Read the model definition and answer for the solid it produces. Units are mm, in the model's axes. A direction names the side the tool comes from. Give positions to 0.01 mm unless a question says otherwise; leave off trailing zeros. Loops run counter-clockwise (first coordinate to the right, second up) from the corner with the lowest first, then second, coordinate; pieces in that order, holes last. Notation, with made-up numbers: (30.25, 50.5) - (50.25, 50.5) arc R14 cw to (50.25, 63.5) - close; hole circle Ø6 at (30, 27.5). An arc over 180 degrees is marked (long way). Use a Markdown table: item, result. Add a question column.
Item 1: A cutting plane is placed at A-A (z = -23). Determine the outline of the cut face in (x, y), plus the area to 3 significant figures.
Item 2: Each of these flat-tipped pins is pushed along its axis until it touches: P1, Ø1, axis at x = 0.5, z = -23, coming from the -Y side; P2, Ø3, axis at y = -2.5, z = -21, coming from the -X side; P3, Ø1.5, axis at x = 2.5, z = -37.5, coming from the -Y side; P4, Ø3, axis at x = -0.5, y = 0, coming from the -Z side. Where does it stop, or does it pass through?
Item 3: A cutting plane is placed at B-B (y = 1.25). Determine the outline of the cut face in (x, z).
Item 4: Which of the six approach directions +Z, -Z, +X, -X, +Y, -Y give full straight-line access (tool end or side, diameter ignored) to faces 1 (the face through (0, 2.79, -45)), 2 (the face through (0, -2.79, -21)), 3 (the face through (0.01, -4.01, -33.61))?
Item 5: A cutting plane is placed at D-D (y = 2.5). Determine the outline of the cut face in (x, z).
Item 6: For a pull along Z with two mould halves and no side action, classify faces 4 (the face through (-0.96, -3.98, -34.5)), 5 (the face through (0, 0, -24.5)), 6 (the face through (-2.427, 1.375, -44.655)) as +Z half, -Z half, draft (parallel to the pull), parting line (faces both ways), or undercut.
Item 7: A cutting plane is placed at C-C (z = -30.5). Determine the outline of the cut face in (x, y), plus the area to 3 significant figures.
Item 8: Consider probe 1 along Y at (x, z) = (-0.25, -45); probe 2 along Z at (x, y) = (1.5, -0.25); probe 3 along X at (y, z) = (-1.5, -23.5). Determine where each line is inside the solid, lowest interval first. Write a range as [from, to].
from build123d import *

# Parameters (mm, degrees)
SKETCH1_W          = 4.5
SKETCH1_H          = 30.85997733
CUT_EXTRUDE1_DEPTH = 7
CUT_EXTRUDE2_DEPTH = 7
CHAMFER1_SIZE      = 0.5
CUT_EXTRUDE3_DEPTH = 1


with BuildPart() as part:
    # Sketch1 → Revolve-Thin1 (revolve)
    with BuildSketch(Plane(origin=(0, 0, 0), x_dir=(1, 0, 0), z_dir=(0, 1, 0))):
        with Locations((2.25, 32.929988665)):
            Rectangle(SKETCH1_W, SKETCH1_H)
    revolve(axis=Axis((0, 0, 0), (0, 0, -1)))

    # Sketch2 → Cut-Extrude1 (cut)
    with BuildSketch(Plane.XY.offset(-17.5)):
        Polygon((1.610807251, 2.79), (-1.610807251, 2.79), (-3.221614502, 0), (-1.610807251, -2.79), (1.610807251, -2.79), (3.221614502, 0), align=None)
    extrude(amount=-CUT_EXTRUDE1_DEPTH, mode=Mode.SUBTRACT)

    # Sketch3 → Cut-Extrude2 (cut)
    with BuildSketch(Plane(origin=(0, 0, -48.35997733), x_dir=(-1, 0, 0), z_dir=(0, 0, -1))):
        Polygon((1.610807251, 2.79), (-1.610807251, 2.79), (-3.221614502, 0), (-1.610807251, -2.79), (1.610807251, -2.79), (3.221614502, 0), align=None)
    extrude(amount=-CUT_EXTRUDE2_DEPTH, mode=Mode.SUBTRACT)

    # Chamfer1
    chamfer1_edges = [part.edges().sort_by_distance(p)[0] for p in [
        (2.416210877, 1.395, -17.5),
        (0, 2.79, -17.5),
        (-2.416210877, 1.395, -17.5),
        (-2.416210877, -1.395, -17.5),
        (0, -2.79, -17.5),
        (2.416210877, -1.395, -17.5),
        (-2.416210877, 1.395, -48.35997733),
        (0, 2.79, -48.35997733),
        (2.416210877, 1.395, -48.35997733),
        (2.416210877, -1.395, -48.35997733),
        (0, -2.79, -48.35997733),
        (-2.416210877, -1.395, -48.35997733),
    ]]
    chamfer(chamfer1_edges, length=CHAMFER1_SIZE)

    # Sketch4 → Cut-Extrude3 (cut)
    with BuildSketch(Plane(origin=(0, -4.5, 0), x_dir=(1, 0, 0), z_dir=(0, 1, 0))):
        with BuildLine():
            Line((-0.735236378, 36.104988665), (-0.183809095, 36.104988665))
            add(Edge.make_bspline(
                [(-0.183809095, 36.104988665), (-0.142887229, 36.104821435), (-0.063984952, 36.104498996), (0.049479088, 36.099913909), (0.153619775, 36.092996425), (0.248313279, 36.083867435), (0.333638661, 36.071201473), (0.40941848, 36.055993448), (0.47613676, 36.039057193), (0.516147477, 36.02331892), (0.534890825, 36.015946197)],
                knots=[0, 0, 0, 0, 0.000122758, 0.000236692, 0.000340599, 0.000435844, 0.000522015, 0.000599225, 0.000667726, 0.000728098, 0.000728098, 0.000728098, 0.000728098], degree=3))
            add(Edge.make_bspline(
                [(0.534890825, 36.015946197), (0.555993425, 36.006429933), (0.597245667, 35.987827142), (0.656357727, 35.95629427), (0.711711569, 35.922324809), (0.762389804, 35.884637999), (0.8094619, 35.84482071), (0.852635966, 35.802494227), (0.891564361, 35.757008969), (0.926655631, 35.709180776), (0.957858636, 35.659071505), (0.984643202, 35.606434054), (1.007803352, 35.551714066), (1.025889509, 35.49431609), (1.04092128, 35.434929127), (1.050643284, 35.373178483), (1.057485172, 35.309272455), (1.058047365, 35.265888615), (1.058333333, 35.243820796)],
                knots=[0, 0, 0, 0, 6.9431e-05, 0.000135726, 0.000200852, 0.000264074, 0.000324989, 0.000385705, 0.00044524, 0.000504393, 0.000563519, 0.000622115, 0.000681412, 0.000741551, 0.000802483, 0.00086501, 0.000928929, 0.000995103, 0.000995103, 0.000995103, 0.000995103], degree=3))
            add(Edge.make_bspline(
                [(1.058333333, 35.243820796), (1.057660809, 35.216664827), (1.056333136, 35.163054546), (1.047657842, 35.083998974), (1.031477343, 35.008136947), (1.009687089, 34.93522949), (0.982690716, 34.864804536), (0.947875359, 34.798087533), (0.907633136, 34.733916018), (0.861157476, 34.67313132), (0.809209736, 34.61517584), (0.749228296, 34.563460322), (0.684531415, 34.51450675), (0.612461254, 34.471597247), (0.53499992, 34.431738139), (0.45038063, 34.397967081), (0.360191554, 34.366801607), (0.296952619, 34.351203721), (0.264583333, 34.343219835)],
                knots=[0, 0, 0, 0, 8.1472e-05, 0.00016084, 0.000238178, 0.00031384, 0.000388957, 0.000464053, 0.000539224, 0.00061593, 0.000693367, 0.000772226, 0.000853128, 0.000936463, 0.001023502, 0.00111421, 0.001209545, 0.001309511, 0.001309511, 0.001309511, 0.001309511], degree=3))
            Line((0.264583333, 34.343219835), (0.997275641, 32.929988665))
            Line((0.997275641, 32.929988665), (0.360621995, 32.929988665))
            Line((0.360621995, 32.929988665), (-0.356805889, 34.313963024))
            Line((-0.356805889, 34.313963024), (-0.41023137, 34.313963024))
            Line((-0.41023137, 34.313963024), (-0.605488782, 32.929988665))
            Line((-0.605488782, 32.929988665), (-1.180448718, 32.929988665))
            Line((-1.180448718, 32.929988665), (-0.735236378, 36.104988665))
        make_face()
        with BuildLine():
            add(Edge.make_bspline(
                [(-0.335817308, 34.843129691), (-0.294894066, 34.843508532), (-0.2166182, 34.84423316), (-0.104827079, 34.849303715), (-0.004219131, 34.857224722), (0.08509361, 34.868749131), (0.16339231, 34.882182886), (0.230523904, 34.899038904), (0.286593934, 34.919072013), (0.332485643, 34.942831056), (0.369661123, 34.970726112), (0.40183809, 35.00049459), (0.428631207, 35.033817084), (0.450737928, 35.070134204), (0.467788114, 35.109521218), (0.480083934, 35.152244969), (0.486882391, 35.198020591), (0.487927508, 35.229595041), (0.488461538, 35.245728849)],
                knots=[0, 0, 0, 0, 0.000122766, 0.000234821, 0.000335651, 0.000425427, 0.000504898, 0.000573853, 0.000632811, 0.000683169, 0.0007282, 0.000771845, 0.000814359, 0.000856026, 0.000899036, 0.000942718, 0.000989043, 0.001037447, 0.001037447, 0.001037447, 0.001037447], degree=3))
            add(Edge.make_bspline(
                [(0.488461538, 35.245728849), (0.487770257, 35.264022258), (0.486429265, 35.299508964), (0.474830234, 35.35062006), (0.454996287, 35.39698474), (0.427122393, 35.438159863), (0.392337213, 35.474465682), (0.349901429, 35.504369125), (0.300298842, 35.527903238), (0.253836196, 35.543471254), (0.210053836, 35.552396101), (0.169082237, 35.558639509), (0.120514754, 35.564294057), (0.064292994, 35.568668304), (0.000652546, 35.571550346), (-0.070576621, 35.574306307), (-0.149461846, 35.575296954), (-0.204585812, 35.575641686), (-0.23341847, 35.575821998)],
                knots=[0, 0, 0, 0, 5.483e-05, 0.000106364, 0.000156221, 0.00020526, 0.000254739, 0.000306272, 0.000360034, 0.000418964, 0.000452769, 0.000493968, 0.000543275, 0.000599421, 0.000663102, 0.000734382, 0.000813258, 0.000899759, 0.000899759, 0.000899759, 0.000899759], degree=3))
            Line((-0.23341847, 35.575821998), (-0.335817308, 34.843129691))
        make_face(mode=Mode.SUBTRACT)
    extrude(amount=CUT_EXTRUDE3_DEPTH, mode=Mode.SUBTRACT)


solid = part.part
Geometry says:
| question | item | result |
|---|---|---|
| 1 | outline | circle Ø9 at (0, 0); hole (-3.22, 0) - (-1.61, -2.79) - (1.61, -2.79) - (3.22, 0) - (1.61, 2.79) - (-1.61, 2.79) - close |
| 1 | area | 36.7 mm² |
| 2 | P1 | y = -4.5 |
| 2 | P2 | x = -4.39 |
| 2 | P3 | y = -4.15 |
| 2 | P4 | z = -41.36 |
| 3 | outline | (-4.32, -48.36) - (-3.08, -48.36) - (-2.5, -47.86) - (-2.5, -41.36) - (2.5, -41.36) - (2.5, -47.86) - (3.08, -48.36) - (4.32, -48.36) - (4.32, -17.5) - (3.08, -17.5) - (2.5, -18) - (2.5, -24.5) - (-2.5, -24.5) - (-2.5, -18) - (-3.08, -17.5) - (-4.32, -17.5) - close |
| 4 | face 1 | -Z |
| 4 | face 2 | +Z |
| 4 | face 3 | -Y |
| 5 | outline | (-3.74, -48.36) - (-2.36, -48.36) - (-1.78, -47.86) - (-1.78, -41.36) - (1.78, -41.36) - (1.78, -47.86) - (2.36, -48.36) - (3.74, -48.36) - (3.74, -17.5) - (2.36, -17.5) - (1.78, -18) - (1.78, -24.5) - (-1.78, -24.5) - (-1.78, -18) - (-2.36, -17.5) - (-3.74, -17.5) - close |
| 6 | face 4 | undercut |
| 6 | face 5 | +Z half |
| 6 | face 6 | draft |
| 7 | outline | circle Ø9 at (0, 0) |
| 7 | area | 63.6 mm² |
| 8 | probe 1 | [-4.49, -2.79], [2.79, 4.49] |
| 8 | probe 2 | [-41.36, -24.5] |
| 8 | probe 3 | [-4.24, -2.36], [2.36, 4.24] |
